CAD build for the part. Positions are in the model's coordinates, mm. A direction names the side the tool comes from. Coordinates: 2 decimals unless noted, no trailing zeros. Order: outer loops, then holes, each group sorted by start corner. A loop starts at its lowest first (then second) coordinate and runs counter-clockwise, first axis right, second up. Notation, with made-up numbers: M 63,-37 L 93,-37 A21 cw 93,-2 Z; hole C -2,18 d4. An arc over 180 degrees is marked long. One line per item, written item: value.
from build123d import *

# Parameters (mm, degrees)
FILLET1_R          = 2
SKETCH3_R          = 2.5
CUT_EXTRUDE1_DEPTH = 6
SKETCH4_R          = 2
CUT_EXTRUDE2_DEPTH = 1.8


with BuildPart() as part:
    # Sketch2 → Revolve2 (revolve)
    with BuildSketch(Plane.XY):
        Polygon((0, -5.7), (0, 5.7), (2.45, 5.7), (2.45, 3.9), (5.1, 3.9), (5.1, -4.6), (3.489000018, -4.6), (3.489000018, -5.7), align=None)
    revolve(axis=Axis((0, -5.7, 0), (0, 1, 0)))

    # Fillet1
    # the kernel refuses this fillet: 2 mm, written as the material it takes off along each edge
    with BuildSketch(Plane(origin=(0, -4.6, 0), x_dir=(1, 0, 0), z_dir=(0, 0, 1))) as fillet1_piece_1:
        with BuildLine():
            CenterArc((3.1, 1.961805033), FILLET1_R, 281.215517004, 78.784482996)
            Line((3.489000018, 0), (3.496780019, -0.039236101))
            ThreePointArc((3.496780019, -0.039236101), (4.294500009, -0.04), (5.1, -0.04))
            Line((5.1, -0.04), (5.14, 0))
            Line((5.14, 0), (5.14, 1.961805033))
            Line((5.14, 1.961805033), (5.1, 1.961805033))
        make_face()
    revolve(axis=Axis((0, -4.6, 0), (0, 1, 0)), mode=Mode.SUBTRACT)
    with BuildSketch(Plane(origin=(0, 3.9, 0), x_dir=(1, 0, 0), z_dir=(0, 0, 1))) as fillet1_piece_2:
        with BuildLine():
            CenterArc((5.1 - FILLET1_R, -FILLET1_R), FILLET1_R, 360, 90)
            Line((5.1, -FILLET1_R), (5.1 + FILLET1_R * 0.02, -FILLET1_R))
            Line((5.1 + FILLET1_R * 0.02, -FILLET1_R), (5.1 + FILLET1_R * 0.02, FILLET1_R * 0.02))
            Line((5.1 + FILLET1_R * 0.02, FILLET1_R * 0.02), (5.1 - FILLET1_R, FILLET1_R * 0.02))
            Line((5.1 - FILLET1_R, FILLET1_R * 0.02), (5.1 - FILLET1_R, 0))
        make_face()
    revolve(axis=Axis((0, 3.9, 0), (0, 1, 0)), mode=Mode.SUBTRACT)

    # Sketch3 → Cut-Extrude1 (cut)
    with BuildSketch(Plane.XZ.offset(5.7)):
        Circle(SKETCH3_R)
    extrude(amount=-CUT_EXTRUDE1_DEPTH, mode=Mode.SUBTRACT)

    # Sketch4 → Cut-Extrude2 (cut)
    with BuildSketch(Plane(origin=(0, 5.7, 0), x_dir=(1, 0, 0), z_dir=(0, 1, 0))):
        with Locations(Location((0, 0, 0), (0, 0, 180))):
            Circle(SKETCH4_R)
    extrude(amount=-CUT_EXTRUDE2_DEPTH, mode=Mode.SUBTRACT)


solid = part.part
Q1. Mould opens along Z. For faces 1 (the face through (-0.54, -2.74, -2.44)), 2 (the face through (2.4, -0.4, 4.5)), 3 (the face through (2, -5.7, 2)) say: released by +Z, released by -Z, zero draft, split by the parting line, or undercut.
Recorded:
face 1: undercut
face 2: split by the parting line
face 3: zero draft
Q2. Pin check, flat tips, straight feed: pin 1 Ø1.5 at (x, y) = (2.5, 1.5) entering from +Z; pin 2 Ø5 at (x, z) = (1, 1) entering from +Y; pin 3 Ø3 at (x, z) = (0, 0) entering from -Y; pin 4 Ø2 at (x, z) = (4, 0) entering from +Y. Stop position of each tip, or through.
Recorded:
pin 1: stops at z = 4.79
pin 2: stops at y = 5.7
pin 3: stops at y = 0.3
pin 4: stops at y = 3.9
Q3. Slice it at D-D (y = 2.5). List the corners of the cut face in (x, z).
Recorded:
outline: C 0,0 d10.02
Q4. Slice it at A-A (x = 0). List the corners of the cut face in (y, z), plus the area to 3 significant figures.
Recorded:
outline: M -5.7,-3.49 L -4.6,-3.49 A2 ccw -2.64,-5.1 L 1.9,-5.1 A2 ccw 3.9,-3.1 L 3.9,-2.45 L 5.7,-2.45 L 5.7,-2 L 3.9,-2 L 3.9,2 L 5.7,2 L 5.7,2.45 L 3.9,2.45 L 3.9,3.1 A2 ccw 1.9,5.1 L -2.64,5.1 A2 ccw -4.6,3.49 L -5.7,3.49 L -5.7,2.5 L 0.3,2.5 L 0.3,-2.5 L -5.7,-2.5 Z
area: 62.7 mm^2
Q5. Which spindle directions (+Z, -Z, +X, -X, +Y, -Y) get a long thin tool onto all of the face, cutting with end or side? Do faces 4 (the face through (0, 5, -2)), 5 (the face through (0, 0.3, 0)), 6 (the face through (1, 5.7, 2)). Say none if no direction does.
Recorded:
face 4: +Y
face 5: -Y
face 6: +Z, -Z, +X, -X, +Y
Q6. Slice it at C-C (y = -0.5). List the corners of the cut face in (x, z), plus the area to 3 significant figures.
Recorded:
outline: C 0,0 d10.2; hole C 0,0 d5
area: 62.1 mm^2
Q7. Drill centre lines: line 1 along Z through (x, y) = (0, -1.45); line 2 along Z through (x, y) = (0, 5.3); line 3 along Y through (x, z) = (-2.75, 0.25). Where is each one in solid material? Low to high.
Recorded:
line 1: z = -5.1 to -2.5, 2.5 to 5.1
line 2: z = -2.45 to -2, 2 to 2.45
line 3: y = -5.7 to 3.9
Q8. Slice it at B-B (z = 0). List the corners of the cut face in (x, y).
Recorded:
outline: M -5.1,-2.64 A2 ccw -3.49,-4.6 L -3.49,-5.7 L -2.5,-5.7 L -2.5,0.3 L 2.5,0.3 L 2.5,-5.7 L 3.49,-5.7 L 3.49,-4.6 A2 ccw 5.1,-2.64 L 5.1,1.9 A2 ccw 3.1,3.9 L 2.45,3.9 L 2.45,5.7 L 2,5.7 L 2,3.9 L -2,3.9 L -2,5.7 L -2.45,5.7 L -2.45,3.9 L -3.1,3.9 A2 ccw -5.1,1.9 Z
